from build123d import *

# Parameters (mm, degrees)
F1_DEPTH       = 25.4
F4_D           = 6.35
F4_DEPTH       = 12.7
F4_CSINK_D     = 13.4874
F4_CSINK_ANGLE = 82
F5_D           = 6.35
F5_DEPTH       = 12.7
F6_R           = 2.54
F7_R           = 2.54


with BuildPart() as f1:
    # F0 (on Front) → F1 (new body)
    with BuildSketch(Plane.XZ):
        Polygon((50.8, 6.35), (0, 6.35), (0, -44.45), (6.35, -44.45), (6.35, 0), (44.45, 0), (44.45, -95.25), (50.8, -95.25), align=None)
    extrude(amount=-F1_DEPTH)

    # F4
    with Locations(Plane.YZ.offset(50.8)):
        with Locations((12.7, -19.05)):
            CounterSinkHole(F4_D / 2, F4_CSINK_D / 2, depth=F4_DEPTH, counter_sink_angle=F4_CSINK_ANGLE)

    # F5
    with Locations(Plane.XY.offset(6.35)):
        with Locations((25.4, 12.7)):
            Hole(F5_D / 2, depth=F5_DEPTH)

    # F6
    f6_edges = [f1.edges().sort_by_distance(p)[0] for p in [
        (0, 12.7, 6.35),
        (50.8, 12.7, 6.35),
    ]]
    fillet(f6_edges, radius=F6_R)

    # F7
    f7_edges = [f1.edges().sort_by_distance(p)[0] for p in [
        (50.8, 12.7, -95.25),
        (6.35, 12.7, -44.45),
        (0, 12.7, -44.45),
    ]]
    fillet(f7_edges, radius=F7_R)


solid = f1.part
Design review of the part built by this model. Coordinates are the model's own, in mm. A direction names the side the tool comes from. Coordinates: 2 decimals unless noted, no trailing zeros. Order: outer loops, then holes, each group sorted by start corner. A loop starts at its lowest first (then second) coordinate and runs counter-clockwise, first axis right, second up. Notation, with made-up numbers: (50, 56) -> (101, 56) arc R4 ccw to (101, 61) -> close; hole circle Ø6 at (20, 2.5). An arc over 180 degrees is marked (long way). Use one line per item in the form item = value. Start each with the question number.
(1) For faces 1 (the flat face through (0, 13, -19)), 2 (the flat face through (44.45, 13, -47)), list the 3-axis set-ups (+Z, -Z, +X, -X, +Y, -Y) from which the entire face can be reached by the end or side of a thin tool; tool diameter is ignored.
(2) For probe 1 along X at (y, z) = (7.5, -28); probe 2 along Y at (x, z) = (46, -19); probe 3 along Z at (x, y) = (36, 22), list the stretches that pass through material, from the lowest coordinate up.
(3) Add section B-B on z = -40. State the section outline as (x, y) points, plus the area to 3 significant figures.
(4) Add section D-D on z = -19.05. State the section outline as (x, y) points (3 decimals), plus the area to 3 significant figures.
(5) Add section A-A on x = 25.4. State the section outline as (y, z) points (3 decimals), plus the area to 3 significant figures.
(6) The part is to be moulded in two halves that separate along X. For faces 3 (the flat face through (50.8, 13, -45)), 4 (the cylindrical face through (45.56, 9.67, -18.1)), 5 (the cylindrical face through (5.586, 12.878, -43.726)), say which applies: +X half, -X half, draft (parallel to the pull), parting line (faces both ways), or undercut.
(7) Insertion check: pin 1 (1 mm diameter, centred on x = 7.5, z = -26, fed in from +Y); pin 2 (8 mm diameter, centred on x = 22.5, y = 22, fed in from -Z); pin 3 (12.5 mm diameter, centred on y = 13, z = -50, fed in from -X). Each pin has a flat end and moves straight along its axis. Give the tip position at first contact, or say it passes through.
(8) Add section C-C on y = 12.7. State the section outline as (x, z) points (3 decimals), plus the area to 3 significant figures.
Answer block:
q1.face_1 = +Z, -Z, -X, +Y, -Y
q1.face_2 = -Z, +Y, -Y
q2.probe_1 = 0 to 6.35, 44.45 to 50.8
q2.probe_2 = 0 to 9.53, 15.87 to 25.4
q2.probe_3 = 0 to 6.35
q3.outline = (0, 0) -> (6.35, 0) -> (6.35, 25.4) -> (0, 25.4) -> close; (44.45, 0) -> (50.8, 0) -> (50.8, 25.4) -> (44.45, 25.4) -> close
q3.area = 323 mm²
q4.outline = (0, 0) -> (6.35, 0) -> (6.35, 25.4) -> (0, 25.4) -> close; (44.45, 0) -> (50.8, 0) -> (50.8, 5.956) -> (46.695, 9.525) -> (44.45, 9.525) -> close; (44.45, 15.875) -> (46.695, 15.875) -> (50.8, 19.444) -> (50.8, 25.4) -> (44.45, 25.4) -> close
q4.area = 268 mm²
q5.outline = (0, 0) -> (9.525, 0) -> (9.525, 6.35) -> (0, 6.35) -> close; (15.875, 0) -> (25.4, 0) -> (25.4, 6.35) -> (15.875, 6.35) -> close
q5.area = 121 mm²
q6.face_3 = +X half
q6.face_4 = draft
q6.face_5 = undercut
q7.pin_1 = through
q7.pin_2 = 0
q7.pin_3 = 0.79
q8.outline = (0, -41.91) arc R2.54 ccw to (2.54, -44.45) -> (3.81, -44.45) arc R2.54 ccw to (6.35, -41.91) -> (6.35, 0) -> (22.225, 0) -> (22.225, 6.35) -> (2.54, 6.35) arc R2.54 ccw to (0, 3.81) -> close; (28.575, 0) -> (44.45, 0) -> (44.45, -15.875) -> (46.695, -15.875) -> (50.8, -12.306) -> (50.8, 3.81) arc R2.54 ccw to (48.26, 6.35) -> (28.575, 6.35) -> close; (44.45, -95.25) -> (48.26, -95.25) arc R2.54 ccw to (50.8, -92.71) -> (50.8, -25.794) -> (46.695, -22.225) -> (44.45, -22.225) -> close
q8.area = 1,110 mm²
